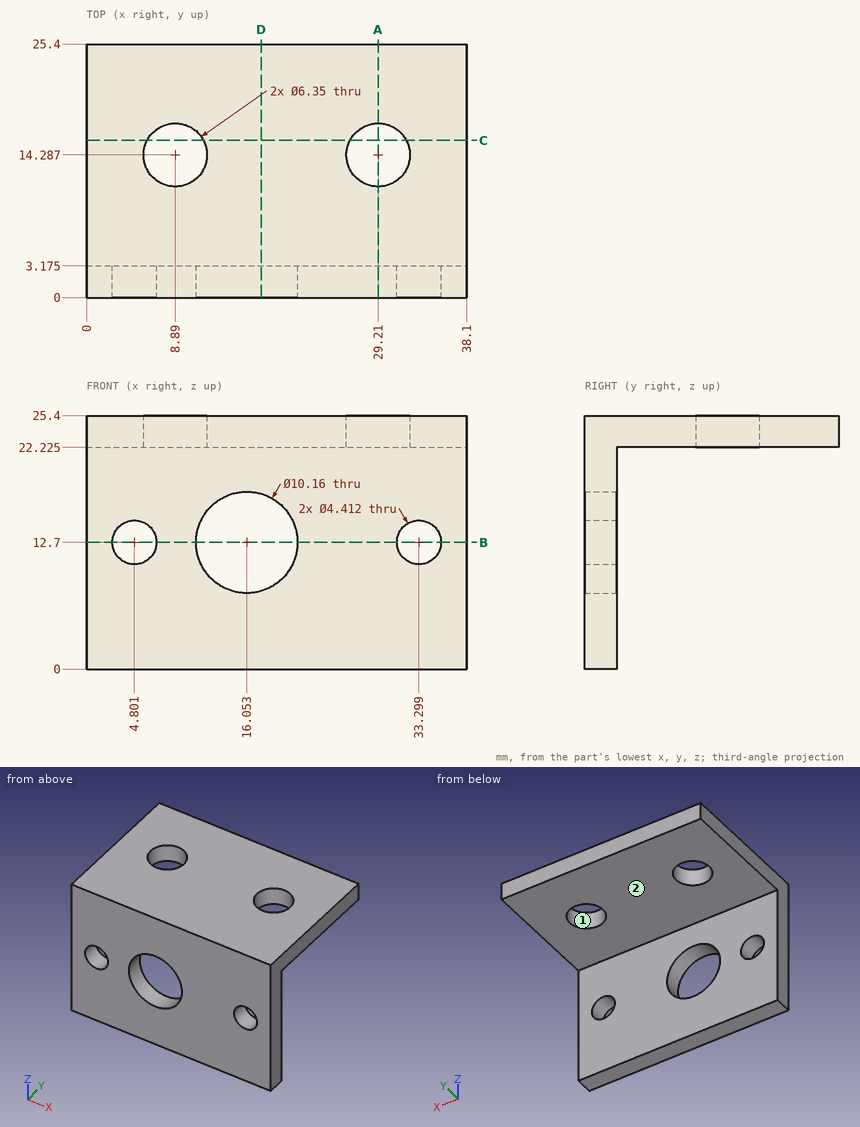
Geometry check sheet. Reference: drawing and pictorial views, mm from the part's lowest x, y, z. A direction names the side the tool comes from. Coordinates: 2 decimals unless noted, no trailing zeros. Order: outer loops, then holes, each group sorted by start corner. A loop starts at its lowest first (then second) coordinate and runs counter-clockwise, first axis right, second up. Notation, with made-up numbers: (65, -18) - (73, -18) arc R16 cw to (73, 5) - close; hole circle Ø6 at (34.5, 47). An arc over 180 degrees is marked (long way). Answer in a Markdown table with one row per item. Add a question column.
1) Cross-section at A-A, the plane x = 29.21. Record the cut outline in (y, z) (1 decimal).
2) Material ranges on line 1 along X through (y, z) = (1.85, 12.7) (1 decimal); line 2 along Y through (x, z) = (8.89, 22.95); line 3 along Y through (x, z) = (32.5, 18.5) (1 decimal), recorded low to high. Write a range as [from, to].
3) Gauge pin test, flat ends, axial feed: P1, Ø6, axis at x = 7, y = 14, coming from the -Z side (1 decimal); P2, Ø3, axis at x = 25, z = 13, coming from the -Y side; P3, Ø9, axis at x = 16.05, z = 12.7, coming from the -Y side; P4, Ø5, axis at x = 33.3, z = 12.7, coming from the +Y side (1 decimal). Record the tip position at first contact, or that the pin passes through.
4) Set-up check for the marked faces 1 and 2: record each of +Z, -Z, +X, -X, +Y, -Y from which the full face is reachable in a straight line by a thin tool's end or side.
5) Cross-section at D-D, the plane x = 17.5. Record the cut outline in (y, z) (1 decimal), then the cut area to 3 significant figures.
6) Cross-section at C-C, the plane y = 15.75. Record the cut outline in (x, z) (1 decimal).
7) Cross-section at B-B, the plane z = 12.7. Record the cut outline in (x, y) (1 decimal).
Check result:
| question | item | result |
|---|---|---|
| 1 | outline | (0, 0) - (3.2, 0) - (3.2, 22.2) - (11.1, 22.2) - (11.1, 25.4) - (0, 25.4) - close; (17.5, 22.2) - (25.4, 22.2) - (25.4, 25.4) - (17.5, 25.4) - close |
| 2 | line 1 | x = [0, 2.6], [7, 11], [21.1, 31.1], [35.5, 38.1] |
| 2 | line 2 | y = [0, 11.11], [17.46, 25.4] |
| 2 | line 3 | y = [0, 3.2] |
| 3 | P1 | stops at z = 22.2 |
| 3 | P2 | stops at y = 0 |
| 3 | P3 | passes through |
| 3 | P4 | stops at y = 3.2 |
| 4 | face 1 | +Z, -Z |
| 4 | face 2 | -Z, +X, -X, +Y |
| 5 | outline | (0, 0) - (3.2, 0) - (3.2, 7.8) - (0, 7.8) - close; (0, 17.6) - (3.2, 17.6) - (3.2, 22.2) - (25.4, 22.2) - (25.4, 25.4) - (0, 25.4) - close |
| 5 | area | 120 mm² |
| 6 | outline | (0, 22.2) - (6.1, 22.2) - (6.1, 25.4) - (0, 25.4) - close; (11.7, 22.2) - (26.4, 22.2) - (26.4, 25.4) - (11.7, 25.4) - close; (32, 22.2) - (38.1, 22.2) - (38.1, 25.4) - (32, 25.4) - close |
| 7 | outline | (0, 0) - (2.6, 0) - (2.6, 3.2) - (0, 3.2) - close; (7, 0) - (11, 0) - (11, 3.2) - (7, 3.2) - close; (21.1, 0) - (31.1, 0) - (31.1, 3.2) - (21.1, 3.2) - close; (35.5, 0) - (38.1, 0) - (38.1, 3.2) - (35.5, 3.2) - close |
